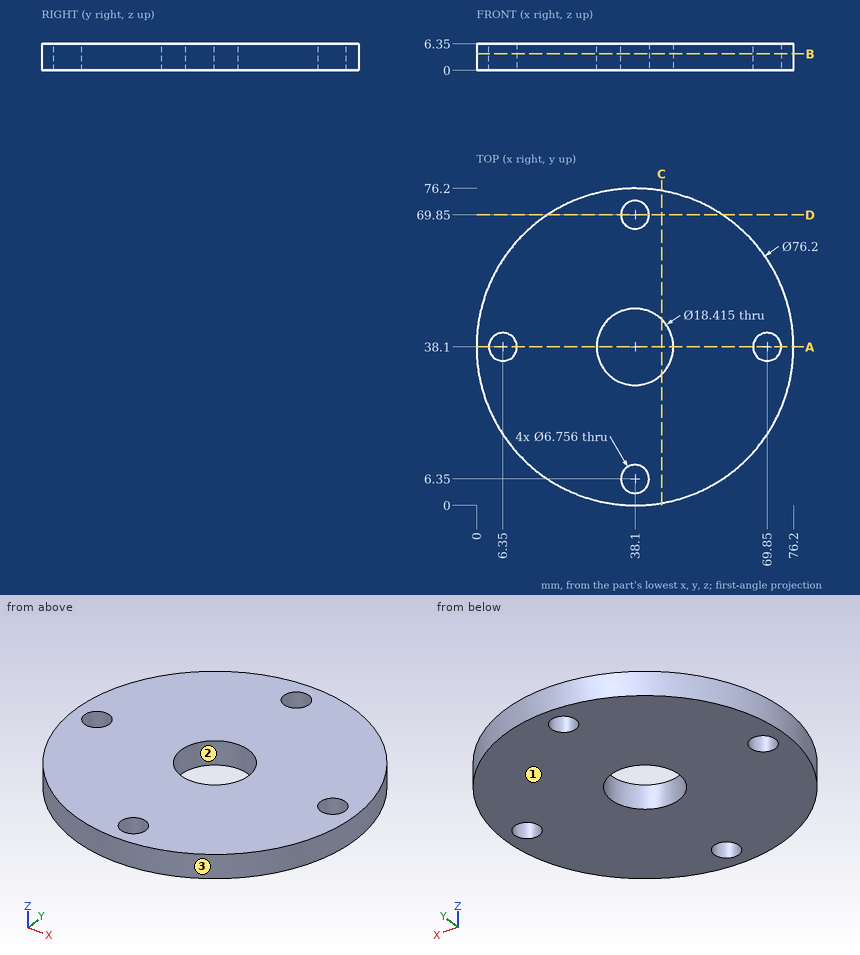
Here's the drawing with two shaded views (mm, measured from the low corner). I have some questions. Coordinates: 2 decimals unless noted, no trailing zeros. Write each loop counter-clockwise with the first axis right and the second up, starting at its lowest first coordinate (ties: lowest second). Pieces come first, ordered by that corner, then holes.
Item 1: I want a section at B-B on z = 4. Count the separate pieces of the cut face and the enclosed holes in it, and give its area (3 significant figures).
Item 2: If I drill on line 1 (Y direction, x = 38.1, z = 4.25); line 2 (Y direction, x = 35, z = 4) (1 decimal); line 3 (Y direction, x = 72, z = 5.25) (1 decimal), over which ranges is the centre line in solid material (lowest first)?
Item 3: I want a section at C-C on x = 44.5. Write out the boundary of the cut face in (y, z).
Item 4: I want a section at A-A on y = 38.1. Write out the boundary of the cut face in (x, z), and give its area (3 significant figures).
Item 5: I want a section at D-D on y = 69.85. Write out the boundary of the cut face in (x, z).
Item 6: Will this pin go through, and if not, where does the flat tip stop? pin 1 (2 mm diameter, centred on y = 27.5, z = 4, fed in from -X).
Item 7: If we mould it in two halves opening along Y, with no side actions, what happens to the marked faces 1, 2 and 3? For each: +Y half, -Y half, draft (parallel to the pull), parting line (faces both ways), or undercut.
Findings below:
1. separate pieces: 1
1. enclosed holes: 5
1. area: 4,150 mm2
2. line 1: y = 0 to 2.97, 9.73 to 28.89, 47.31 to 66.47, 73.23 to 76.2
2. line 2: y = 0.1 to 5, 7.7 to 29.4, 46.8 to 68.5, 71.2 to 76.1
2. line 3: y = 20.7 to 35.5, 40.7 to 55.5
3. outline: (0.54, 0) - (31.48, 0) - (31.48, 6.35) - (0.54, 6.35) - close; (44.72, 0) - (75.66, 0) - (75.66, 6.35) - (44.72, 6.35) - close
4. outline: (0, 0) - (2.97, 0) - (2.97, 6.35) - (0, 6.35) - close; (9.73, 0) - (28.89, 0) - (28.89, 6.35) - (9.73, 6.35) - close; (47.31, 0) - (66.47, 0) - (66.47, 6.35) - (47.31, 6.35) - close; (73.23, 0) - (76.2, 0) - (76.2, 6.35) - (73.23, 6.35) - close
4. area: 281 mm2
5. outline: (17.04, 0) - (34.72, 0) - (34.72, 6.35) - (17.04, 6.35) - close; (41.48, 0) - (59.16, 0) - (59.16, 6.35) - (41.48, 6.35) - close
6. pin 1: stops at x = 1.23
7. face 1: draft
7. face 2: undercut
7. face 3: parting line
